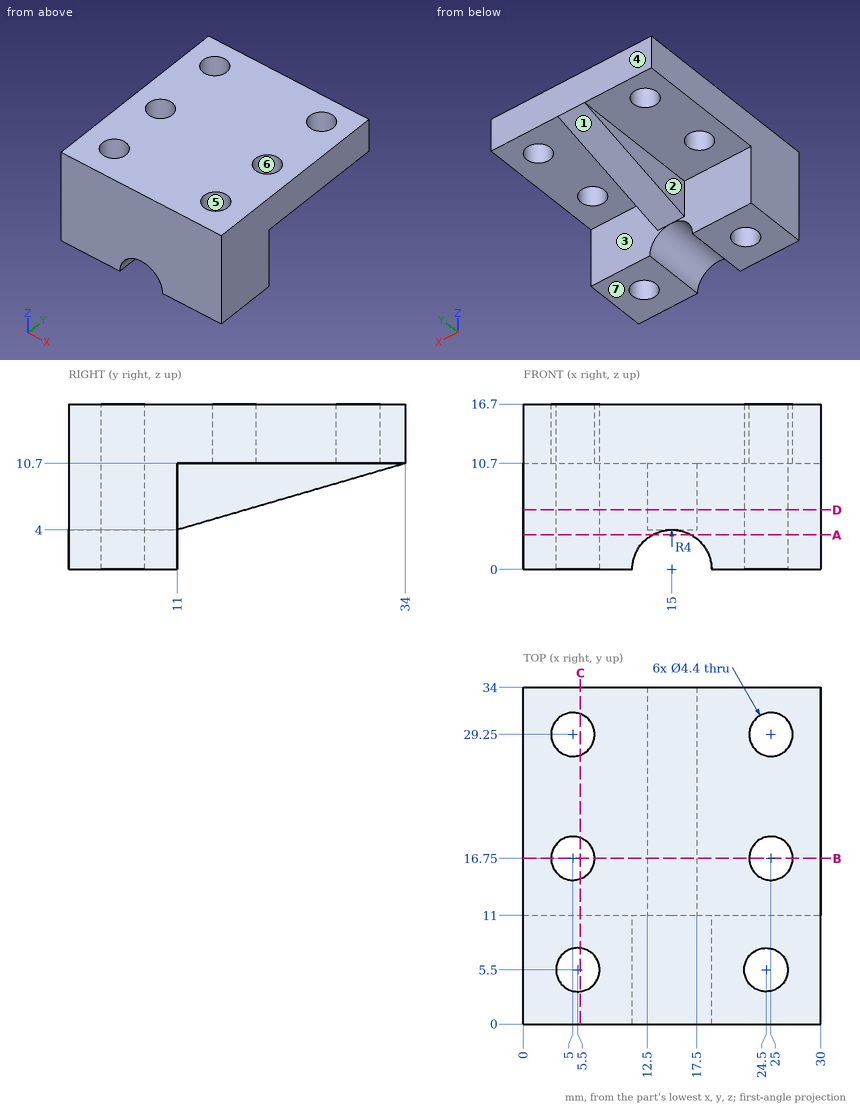
Design review of the part shown in the three views and the two pictorial views. Dimensions are in mm from the part's minimum x, y and z. A direction names the side the tool comes from. Round coordinates to 2 decimals unless told otherwise and drop trailing zeros. Loops run counter-clockwise (first coordinate to the right, second up) from the corner with the lowest first, then second, coordinate; pieces in that order, holes last. Notation, with made-up numbers: (78, 10.5) -> (82, 10.5) arc R30 cw to (82, 40.5) -> close; hole circle Ø1 at (-30, 29.5). An arc over 180 degrees is marked (long way). Answer as a JSON object with one key per item and string values. Group by question number.
1) We need section A-A on z = 3.5. Write out the cut boundary in (x, y).
2) We need section B-B on y = 16.75. Write out the cut boundary in (x, z) (3 decimals), then the cut area to 3 significant figures.
3) For line 1 (X direction, y = 29.5, z = 14); line 2 (Y direction, x = 5, z = 12.5); line 3 (Y direction, x = 24.5, z = 7.75), list the stretches that pass through material, from the lowest coordinate up. Write a range as [from, to].
4) For the marked faces 1, 2 and 3, list the 3-axis set-ups (+Z, -Z, +X, -X, +Y, -Y) from which the entire face can be reached by the end or side of a thin tool; tool diameter is ignored.
5) Mouldability with a two-part tool opening along Y and no side actions: class the marked faces 4, 5, 6 and 7 as released by +Y, released by -Y, zero draft, split by the parting line, or undercut.
6) We need section C-C on x = 5.75. Write out the cut boundary in (y, z).
7) For pin 1 Ø2 at (y, z) = (17, 5) entering from +X; pin 2 Ø5 at (y, z) = (21.5, 6.5) entering from -X; pin 3 Ø3 at (x, y) = (6, 27.5) entering from -Z, all flat-tipped, find the tip position at first contact; note any pin that passes through.
8) We need section D-D on z = 6. Write out the cut boundary in (x, y), then the cut area to 3 significant figures.
Result set:
{
 "1": {"outline": "(0, 0) -> (13.06, 0) -> (13.06, 11) -> (0, 11) -> close; (16.94, 0) -> (30, 0) -> (30, 11) -> (16.94, 11) -> close; hole circle Ø4.4 at (5.5, 5.5); hole circle Ø4.4 at (24.5, 5.5)"},
 "2": {"outline": "(0, 10.7) -> (2.8, 10.7) -> (2.8, 16.7) -> (0, 16.7) -> close; (7.2, 10.7) -> (12.5, 10.7) -> (12.5, 5.675) -> (17.5, 5.675) -> (17.5, 10.7) -> (22.8, 10.7) -> (22.8, 16.7) -> (7.2, 16.7) -> close; (27.2, 10.7) -> (30, 10.7) -> (30, 16.7) -> (27.2, 16.7) -> close", "area": "152 mm²"},
 "3": {"line 1": "[0, 2.81], [7.19, 22.81], [27.19, 30]", "line 2": "[0, 3.36], [7.64, 14.55], [18.95, 27.05], [31.45, 34]", "line 3": "[0, 3.3], [7.7, 11]"},
 "4": {"face 1": "-Z, +X, -X, +Y", "face 2": "-Z, -X, +Y", "face 3": "-Z, +X, +Y"},
 "5": {"face 4": "released by +Y", "face 5": "undercut", "face 6": "undercut", "face 7": "zero draft"},
 "6": {"outline": "(0, 0) -> (3.31, 0) -> (3.31, 16.7) -> (0, 16.7) -> close; (7.69, 0) -> (11, 0) -> (11, 10.7) -> (14.68, 10.7) -> (14.68, 16.7) -> (7.69, 16.7) -> close; (18.82, 10.7) -> (27.18, 10.7) -> (27.18, 16.7) -> (18.82, 16.7) -> close; (31.32, 10.7) -> (34, 10.7) -> (34, 16.7) -> (31.32, 16.7) -> close"},
 "7": {"pin 1": "x = 17.5", "pin 2": "x = 12.5", "pin 3": "z = 10.7"},
 "8": {"outline": "(0, 0) -> (30, 0) -> (30, 11) -> (17.5, 11) -> (17.5, 17.87) -> (12.5, 17.87) -> (12.5, 11) -> (0, 11) -> close; hole circle Ø4.4 at (5.5, 5.5); hole circle Ø4.4 at (24.5, 5.5)", "area": "334 mm²"}
}
